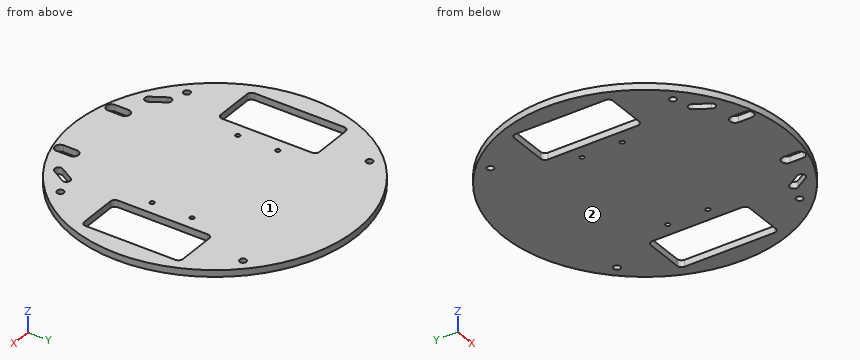
```python
from build123d import *

# Parameters (mm, degrees)
BOSS_EXTRUDE1_OUTLINE_R   = 63.5
BOSS_EXTRUDE1_OUTLINE_R_2 = 1.5
BOSS_EXTRUDE1_OUTLINE_R_3 = 1
BOSS_EXTRUDE1_OUTLINE_W   = 21
BOSS_EXTRUDE1_OUTLINE_H   = 44.3
BOSS_EXTRUDE1_DEPTH       = 3
FILLET1_R                 = 2


# Read off the part's stored shape, not the designer's step: Boss-Extrude1
with BuildPart() as part:
    # Boss-Extrude1 outline → Boss-Extrude1 (new body)
    with BuildSketch(Plane.XY):
        Circle(BOSS_EXTRUDE1_OUTLINE_R)
        with Locations((-41, -41)):
            Circle(BOSS_EXTRUDE1_OUTLINE_R_2, mode=Mode.SUBTRACT)
        with BuildLine():
            Line((-19, -58), (-19, -52))
            ThreePointArc((-19, -52), (-16.7, -49.7), (-14.4, -52))
            Line((-14.4, -52), (-14.4, -58))
            ThreePointArc((-14.4, -58), (-16.7, -60.3), (-19, -58))
        make_face(mode=Mode.SUBTRACT)
        with BuildLine():
            Line((-30.697224362, -50.901387819), (-34.302775638, -44.901387819))
            ThreePointArc((-34.302775638, -44.901387819), (-33.704163457, -42.5), (-31.302775638, -43.098612181))
            Line((-31.302775638, -43.098612181), (-27.697224362, -49.098612181))
            ThreePointArc((-27.697224362, -49.098612181), (-28.295836543, -51.5), (-30.697224362, -50.901387819))
        make_face(mode=Mode.SUBTRACT)
        with Locations((-27.75, -9)):
            Circle(BOSS_EXTRUDE1_OUTLINE_R_3, mode=Mode.SUBTRACT)
        with BuildLine():
            Line((14.4, -58), (14.4, -52))
            ThreePointArc((14.4, -52), (16.7, -49.7), (19, -52))
            Line((19, -52), (19, -58))
            ThreePointArc((19, -58), (16.7, -60.3), (14.4, -58))
        make_face(mode=Mode.SUBTRACT)
        with BuildLine():
            Line((34.302775638, -44.901387819), (30.697224362, -50.901387819))
            ThreePointArc((30.697224362, -50.901387819), (28.295836543, -51.5), (27.697224362, -49.098612181))
            Line((27.697224362, -49.098612181), (31.302775638, -43.098612181))
            ThreePointArc((31.302775638, -43.098612181), (33.704163457, -42.5), (34.302775638, -44.901387819))
        make_face(mode=Mode.SUBTRACT)
        with Locations((41, -41)):
            Circle(BOSS_EXTRUDE1_OUTLINE_R_2, mode=Mode.SUBTRACT)
        with Locations((27.75, -9)):
            Circle(BOSS_EXTRUDE1_OUTLINE_R_3, mode=Mode.SUBTRACT)
        with Locations((-44.25, 0)):
            Rectangle(BOSS_EXTRUDE1_OUTLINE_W, BOSS_EXTRUDE1_OUTLINE_H, mode=Mode.SUBTRACT)
        with Locations((-27.75, 9)):
            Circle(BOSS_EXTRUDE1_OUTLINE_R_3, mode=Mode.SUBTRACT)
        with Locations((-41, 41)):
            Circle(BOSS_EXTRUDE1_OUTLINE_R_2, mode=Mode.SUBTRACT)
        with Locations((27.75, 9)):
            Circle(BOSS_EXTRUDE1_OUTLINE_R_3, mode=Mode.SUBTRACT)
        with Locations((44.25, 0)):
            Rectangle(BOSS_EXTRUDE1_OUTLINE_W, BOSS_EXTRUDE1_OUTLINE_H, mode=Mode.SUBTRACT)
        with Locations((41, 41)):
            Circle(BOSS_EXTRUDE1_OUTLINE_R_2, mode=Mode.SUBTRACT)
    extrude(amount=BOSS_EXTRUDE1_DEPTH)

    # Fillet1
    fillet1_edges = [part.edges().sort_by_distance(p)[0] for p in [
        (-54.75, 22.15, 1.5),
        (-54.75, -22.15, 1.5),
        (-33.75, -22.15, 1.5),
        (-33.75, 22.15, 1.5),
        (33.75, 22.15, 1.5),
        (33.75, -22.15, 1.5),
        (54.75, -22.15, 1.5),
        (54.75, 22.15, 1.5),
    ]]
    fillet(fillet1_edges, radius=FILLET1_R)


solid = part.part
```
Verification items for the finished model (mm, model axes). Face numbers are marked on the shaded views. Coordinates: 2 decimals unless noted, no trailing zeros. Write each loop counter-clockwise with the first axis right and the second up, starting at its lowest first coordinate (ties: lowest second). Pieces come first, ordered by that corner, then holes. Notation, with made-up numbers: M 68.25,47 L 117.25,47 A24 cw 117.25,73 Z; hole C -33,-15.75 d11. An arc over 180 degrees is marked long. Answer as a JSON object with one key per item and string values. Group by question number.
(1) Cross-section at B-B, the plane x = -16.7. Record the cut outline in (y, z).
(2) Cross-section at D-D, the plane y = 13.5. Record the cut outline in (x, z), and give its area (3 significant figures).
(3) Release check for a two-part mould opening along Z. For the marked faces 1 and 2 record: +Z half, -Z half, draft (parallel to the pull), parting line (faces both ways), or undercut.
(4) Material ranges on line 1 (X direction, y = 40.5, z = 0.8); line 2 (Y direction, x = -27.75, z = 2.25); line 3 (X direction, y = -14, z = 1.45), recorded low to high.
(5) Cross-section at A-A, the plane y = 0. Record the cut outline in (x, z).
(6) Gauge pin test, flat ends, axial feed: pin 1 (1.2 mm diameter, centred on x = 27.75, y = 9, fed in from +Z); pin 2 (1.5 mm diameter, centred on x = -41, z = 2, fed in from +Y); pin 3 (1.5 mm diameter, centred on x = 41, z = 1.5, fed in from -Y); pin 4 (1 mm diameter, centred on x = 25.5, z = 1.5, fed in from +Y). Record the tip position at first contact, or that the pin passes through.
(7) Cross-section at C-C, the plane z = 2.45. State how many separate pieces and enclosed holes the cut face has, and give its area (3 significant figures).
Reply:
{
 "1": {"outline": "M -61.26,0 L -60.3,0 L -60.3,3 L -61.26,3 Z; M -49.7,0 L 61.26,0 L 61.26,3 L -49.7,3 Z"},
 "2": {"outline": "M -62.05,0 L -54.75,0 L -54.75,3 L -62.05,3 Z; M -33.75,0 L 33.75,0 L 33.75,3 L -33.75,3 Z; M 54.75,0 L 62.05,0 L 62.05,3 L 54.75,3 Z", "area": "246 mm²"},
 "3": {"face 1": "+Z half", "face 2": "-Z half"},
 "4": {"line 1": "-48.91 to -42.41, -39.59 to 39.59, 42.41 to 48.91", "line 2": "-57.12 to -50.98, -49.01 to -10, -8 to 8, 10 to 57.12", "line 3": "-61.94 to -54.75, -33.75 to 33.75, 54.75 to 61.94"},
 "5": {"outline": "M -63.5,0 L -54.75,0 L -54.75,3 L -63.5,3 Z; M -33.75,0 L 33.75,0 L 33.75,3 L -33.75,3 Z; M 54.75,0 L 63.5,0 L 63.5,3 L 54.75,3 Z"},
 "6": {"pin 1": "through", "pin 2": "y = 49.11", "pin 3": "y = -49.11", "pin 4": "y = 58.37"},
 "7": {"separate pieces": "1", "enclosed holes": "14", "area": "10,600 mm²"}
}
